Study the drawing (mm; zero at the part's minimum x, y, z) and answer. Round coordinates to 2 decimals unless told otherwise and drop trailing zeros. Order: outer loops, then holes, each group sorted by start corner. A loop starts at its lowest first (then second) coordinate and runs counter-clockwise, first axis right, second up. Notation, with made-up numbers: (46, -32) - (51, -32) arc R19 ccw to (51, 3) - close; hole circle Ø10 at (58.5, 1). An arc over 180 degrees is marked (long way). Use one line per item in the form item = value. Start each with the question number.
Q1. The part is cut by section A-A on y = 44.45. Determine the outline of the cut face in (x, z).
Q2. Find the intervals of material crossed by line 1 (Y direction, x = 1.25, z = 4.75); line 2 (Y direction, x = 4.75, z = 2.5); line 3 (Y direction, x = 2.75, z = 3.5) (1 decimal), in increasing order. Write a range as [from, to].
Q3. Given P1, Ø2.5, axis at x = 4.572, y = 44.45, coming from the -Z side, flat-ended and moving along its own axis, determine where the tip first touches the part or whether it passes through.
Q4. The part is cut by section D-D on x = 1.25. Determine the outline of the cut face in (y, z).
Q5. The part is cut by section B-B on z = 3. Determine the outline of the cut face in (x, y).
Q6. The part is cut by section C-C on x = 3.5. Determine the outline of the cut face in (y, z).
Q7. For a pull along Y with two mould halves and no side action, classify the marked faces 1, 2 and 3 as +Y half, -Y half, draft (parallel to the pull), parting line (faces both ways), or undercut.
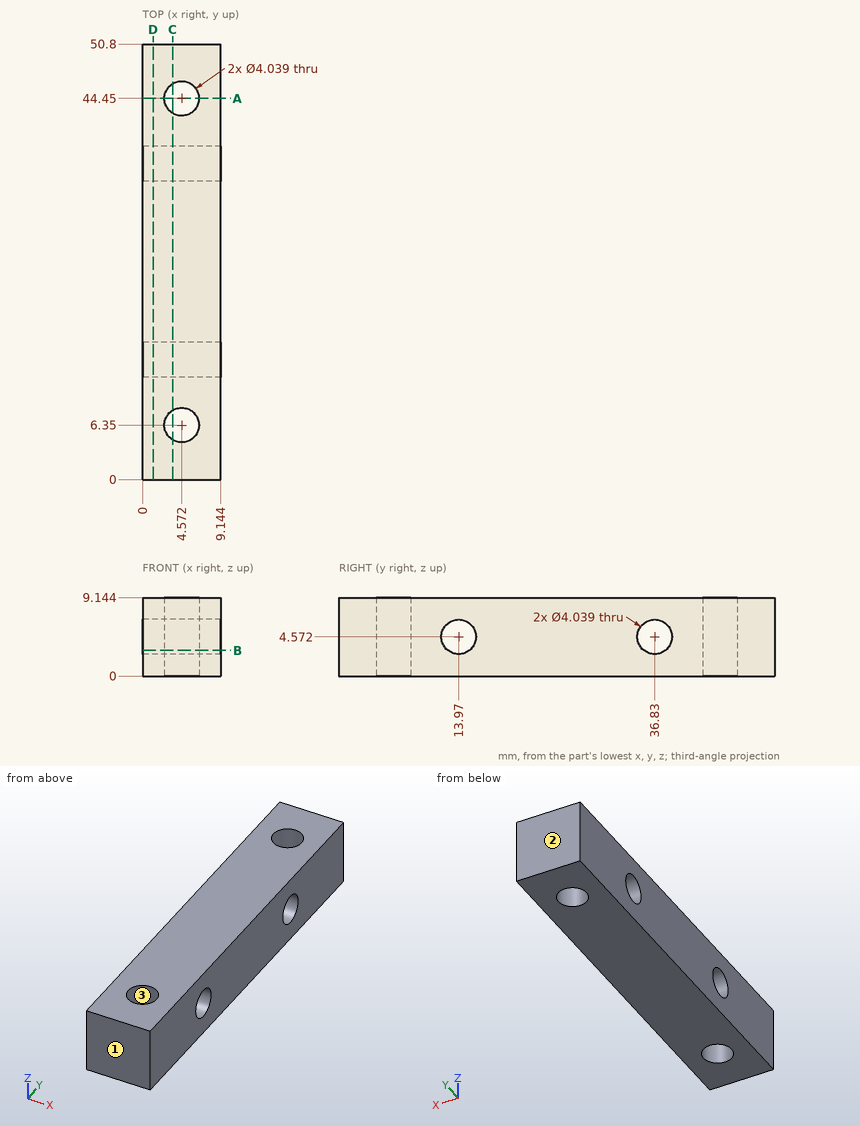
Found:
q1.outline = (0, 0) - (2.55, 0) - (2.55, 9.14) - (0, 9.14) - close; (6.59, 0) - (9.14, 0) - (9.14, 9.14) - (6.59, 9.14) - close
q2.line_1 = [0, 11.96], [15.98, 34.82], [38.84, 50.8]
q2.line_2 = [0, 4.34], [8.36, 42.44], [46.46, 50.8]
q2.line_3 = [0, 5.5], [7.2, 12.3], [15.7, 35.1], [38.5, 43.6], [45.3, 50.8]
q3.P1 = through
q4.outline = (0, 0) - (50.8, 0) - (50.8, 9.14) - (0, 9.14) - close; hole circle Ø4.04 at (13.97, 4.57); hole circle Ø4.04 at (36.83, 4.57)
q5.outline = (0, 0) - (9.14, 0) - (9.14, 12.7) - (0, 12.7) - close; (0, 15.24) - (9.14, 15.24) - (9.14, 35.56) - (0, 35.56) - close; (0, 38.1) - (9.14, 38.1) - (9.14, 50.8) - (0, 50.8) - close; hole circle Ø4.04 at (4.57, 6.35); hole circle Ø4.04 at (4.57, 44.45)
q6.outline = (0, 0) - (4.64, 0) - (4.64, 9.14) - (0, 9.14) - close; (8.06, 0) - (42.74, 0) - (42.74, 9.14) - (8.06, 9.14) - close; (46.16, 0) - (50.8, 0) - (50.8, 9.14) - (46.16, 9.14) - close; hole circle Ø4.04 at (13.97, 4.57); hole circle Ø4.04 at (36.83, 4.57)
q7.face_1 = -Y half
q7.face_2 = +Y half
q7.face_3 = undercut
